Autodesk Inventor part; units mm, degrees
ref_plane "YZ Plane" through (0, 0, 0) normal (1, 0, 0) x (0, 1, 0)
ref_plane "XZ Plane" through (0, 0, 0) normal (0, 1, 0) x (-1, 0, 0)
ref_plane "XY Plane" through (0, 0, 0) normal (0, 0, 1) x (1, 0, 0)
sketch "Sketch1" plane through (0, 0, 0) normal (0, 1, 0) x (-1, 0, 0)
  line L0 (6.4, 0) -> (3.2, -5.5426)
  line L1 (3.2, -5.5426) -> (-3.2, -5.5426)
  line L2 (-3.2, -5.5426) -> (-6.4, 0)
  line L3 (-6.4, 0) -> (-3.2, 5.5426)
  line L4 (-3.2, 5.5426) -> (3.2, 5.5426)
  line L5 (3.2, 5.5426) -> (6.4, 0)
  point P0 (0, 0)
  dimension "d1" = 6.4
extrude "Extrusion1" add sketch "Sketch1" along normal blind 18.5
sketch "Sketch2" plane through (0, 18.5, 0) normal (0, 1, 0) x (1, 0, 0)
  circle A0 centre (0, 0) radius 1.25
  dimension "d4" = 2.5
extrude "Extrusion2" cut sketch "Sketch2" against normal blind 8
sketch "Sketch3" plane through (0, 0, 0) normal (0, -1, 0) x (1, 0, 0)
  circle A0 centre (0, 0) radius 1.5
  dimension "d7" = 3
extrude "Extrusion3" cut sketch "Sketch3" against normal blind 8.6
Verification items for the finished model (mm, model axes). A direction names the side the tool comes from. Round coordinates to 2 decimals unless told otherwise and drop trailing zeros. Loops run counter-clockwise (first coordinate to the right, second up) from the corner with the lowest first, then second, coordinate; pieces in that order, holes last. Notation, with made-up numbers: (36.25, -18) - (43.25, -18) arc R18 cw to (43.25, -14) - close; hole circle Ø2 at (-17.5, -17). An arc over 180 degrees is marked (long way). Use one line per item in the form item = value.
1. Gauge pin test, flat ends, axial feed: pin 1 Ø6 at (y, z) = (11, -4) entering from +X; pin 2 Ø1 at (y, z) = (10.5, 3.5) entering from +X; pin 3 Ø6 at (y, z) = (9, -1) entering from -X. Record the tip position at first contact, or that the pin passes through.
A:
pin_1 = 5.82
pin_2 = 4.67
pin_3 = -6.4
2. Scan lines: probe 1 along Z at (x, y) = (0, 12.5); probe 2 along Z at (x, y) = (0, 8); probe 3 along Y at (x, z) = (0.5, -0.5). Record each from-to range of solid material in increasing order.
A:
probe_1 = -5.54 to -1.25, 1.25 to 5.54
probe_2 = -5.54 to -1.5, 1.5 to 5.54
probe_3 = 8.6 to 10.5
3. Section check D-D on y = 11.5. Record the cut outline in (x, z), and give its area (3 significant figures).
A:
outline = (-6.4, 0) - (-3.2, -5.54) - (3.2, -5.54) - (6.4, 0) - (3.2, 5.54) - (-3.2, 5.54) - close; hole circle Ø2.5 at (0, 0)
area = 102 mm²
4. Section check C-C on x = 0. Record the cut outline in (y, z), and give its area (3 significant figures).
A:
outline = (0, -5.54) - (18.5, -5.54) - (18.5, -1.25) - (10.5, -1.25) - (10.5, 1.25) - (18.5, 1.25) - (18.5, 5.54) - (0, 5.54) - (0, 1.5) - (8.6, 1.5) - (8.6, -1.5) - (0, -1.5) - close
area = 159 mm²
5. Section check B-B on z = 0.5. Record the cut outline in (x, y).
A:
outline = (-6.11, 0) - (-1.41, 0) - (-1.41, 8.6) - (1.41, 8.6) - (1.41, 0) - (6.11, 0) - (6.11, 18.5) - (1.15, 18.5) - (1.15, 10.5) - (-1.15, 10.5) - (-1.15, 18.5) - (-6.11, 18.5) - close
6. Access from +Z, -Z, +X, -X, +Y, -Y to the whole of each face (thin tool, end or side, straight path). Record for faces 5 (the flat face through (0, 9, 5.543)), 6 (the cylindrical face through (-1.5, 4.24, 0.07)).
A:
face_5 = +Z, +X, -X, +Y, -Y
face_6 = -Y
7. Section check A-A on y = 1.5. Record the cut outline in (x, z), and give its area (3 significant figures).
A:
outline = (-6.4, 0) - (-3.2, -5.54) - (3.2, -5.54) - (6.4, 0) - (3.2, 5.54) - (-3.2, 5.54) - close; hole circle Ø3 at (0, 0)
area = 99.3 mm²
8. Draft check along X on faces 1 (the cylindrical face through (-0.27, 14.56, 1.22)), 2 (the flat face through (0, 10.5, 0)), 3 (the flat face through (4.778, 9.12, -2.81)), 4 (the flat face through (-4.822, 9.12, -2.733)). Enter one of: pulls with the +X half, pulls with the -X half, needs draft (parallel to the pull), parting line crosses it, or undercut.
A:
face_1 = undercut
face_2 = undercut
face_3 = pulls with the +X half
face_4 = pulls with the -X half
